Can you work these out from the model? Positions are in its coordinate system, mm. Face numbers are marked on the shaded views. Give positions to 0.01 mm unless a question says otherwise; leave off trailing zeros. Loops run counter-clockwise (first coordinate to the right, second up) from the corner with the lowest first, then second, coordinate; pieces in that order, holes last. Notation, with made-up numbers: (-12, -26.75) -> (21, -26.75) arc R22 ccw to (21, -16.75) -> close; hole circle Ø3 at (-36, 74.25). An arc over 180 degrees is marked (long way). Use CSV: the item, a comma, the result in double quotes.
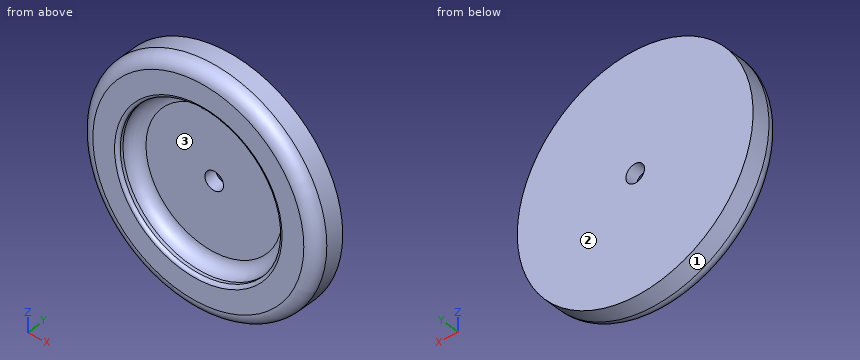
Autodesk Inventor part; units mm, degrees
ref_plane "YZ Plane" through (0, 0, 0) normal (1, 0, 0) x (0, 1, 0)
ref_plane "XZ Plane" through (0, 0, 0) normal (0, 1, 0) x (-1, 0, 0)
ref_plane "XY Plane" through (0, 0, 0) normal (0, 0, 1) x (1, 0, 0)
sketch "Sketch1" plane through (0, 0, 0) normal (0, 0, 1) x (1, 0, 0)
  line L0 (0, 0) -> (19, 0)
  line L1 (0, 0) -> (0, -2)
  line L2 (0, -2) -> (13, -2)
  line L3 (13, -2) -> (13, -5)
  line L4 (13, -5) -> (17, -5)
  line L5 (19, -3) -> (19, 0)
  line L6 (1.5, 0) -> (1.5, -2)
  arc A0 (17, -5) -> (19, -3) centre (17, -3) ccw
  point P0 (19, -5)
  dimension "d5" = 19
  dimension "d12" = 2
  dimension "d16" = 5
  dimension "d17" = 1.5
  dimension "d23" = 2
  dimension "d24" = 90
  dimension "d25" = 4
revolve "Revolution1" add sketch "Sketch1" angle 360 about axis through (0, 0, 0) along (0, -1, 0) contours L0 L5 A0 L4 L3 L2 L6
fillet "Fillet2" radius 0.5 1 edges at (-13, -5, 0)
fillet "Fillet3" radius 2 1 edges at (-13, -2, 0)
properties part number "Seal_M_TPU"
(1) We'd pull the mould along X, two halves only. Please class the marked faces 1, 2 and 3: released by +X, released by -X, zero draft, split by the parting line, or undercut.
Answer sheet:
face 1,"split by the parting line"
face 2,"zero draft"
face 3,"undercut"
(2) If we section it at A-A, the plane z = 0: Write out the boundary of the cut face in (x, y), then the cut area to 3 significant figures.
Answer sheet:
outline,"(-19, -3) arc R2 ccw to (-17, -5) -> (-13.5, -5) arc R0.5 ccw to (-13, -4.5) -> (-13, -4) arc R2 cw to (-11, -2) -> (-1.5, -2) -> (-1.5, 0) -> (-19, 0) -> close; (1.5, -2) -> (11, -2) arc R2 cw to (13, -4) -> (13, -4.5) arc R0.5 ccw to (13.5, -5) -> (17, -5) arc R2 ccw to (19, -3) -> (19, 0) -> (1.5, 0) -> close"
area,"106 mm2"
(3) If we section it at C-C, the plane y = -1.5: Write out the boundary of the cut face in (x, z).
Answer sheet:
outline,"circle Ø38 at (0, 0); hole circle Ø3 at (0, 0)"
(4) If we section it at B-B, the plane x = 0: Write out the boundary of the cut face in (y, z), then the cut area to 3 significant figures.
Answer sheet:
outline,"(-5, -17) arc R2 ccw to (-3, -19) -> (0, -19) -> (0, -1.5) -> (-2, -1.5) -> (-2, -11) arc R2 cw to (-4, -13) -> (-4.5, -13) arc R0.5 ccw to (-5, -13.5) -> close; (-5, 13.5) arc R0.5 ccw to (-4.5, 13) -> (-4, 13) arc R2 cw to (-2, 11) -> (-2, 1.5) -> (0, 1.5) -> (0, 19) -> (-3, 19) arc R2 ccw to (-5, 17) -> close"
area,"106 mm2"
(5) If I drill on L1, parallel to Z at x = 0, y = -0.7; L2, parallel to Y at x = -8.5, z = 5; L3, parallel to Z at x = 0, y = -4.05, over which ranges is the centre line in solid material (lowest first)? Write a range as from..to.
Answer sheet:
L1,"z = -19..-1.5, 1.5..19"
L2,"y = -2..0"
L3,"z = -18.7..-13, 13..18.7"
(6) Will these pins go through, and if not, where does the flat tip stop? pin 1 Ø2 at (x, z) = (-1.5, 3.5) entering from +Y; pin 2 Ø2 at (x, y) = (-7, -3.5) entering from -Z; pin 3 Ø3 at (y, z) = (-3, -12.5) entering from -X; pin 4 Ø1.8 at (x, z) = (0, 0) entering from +Y.
Answer sheet:
pin 1,"stops at y = 0"
pin 2,"stops at z = -18"
pin 3,"stops at x = -15.49"
pin 4,"passes through"
